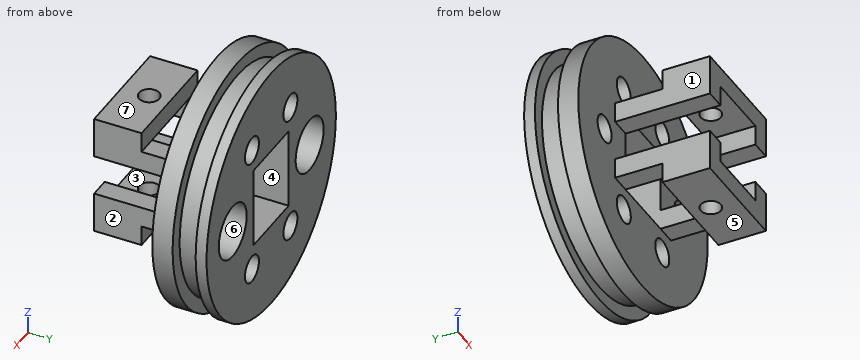
from build123d import *

# Parameters (mm, degrees)
SKETCH_1_R               = 11
EXTRUDE_1_DEPTH          = 9
SKETCH_2_R               = 1
CUT_EXTRUDE_1_DEPTH      = 10
SKETCH_3_R               = 16.549134696
SKETCH_3_R_2             = 9.25
CUT_EXTRUDE_2_DEPTH      = 7
SKETCH_4_W               = 2
SKETCH_4_H               = 1.7
SKETCH_5_W               = 5
SKETCH_5_H               = 6
CUT_EXTRUDE_3_DEPTH      = 7
SKETCH_6_R               = 1.4
CUT_EXTRUDE_4_DEPTH      = 7
PATTERN_CIRCULAR_1_COUNT = 3
PATTERN_CIRCULAR_1_ANGLE = 120
SKETCH_10_R              = 17.755262973
CUT_EXTRUDE_8_DEPTH      = 5
SKETCH_11_R              = 2
CUT_EXTRUDE_9_DEPTH      = 3
SKETCH_12_W              = 1.5
SKETCH_12_H              = 1.5
EXTRUDE_2_DEPTH          = 3.5
SKETCH_14_W              = 1.5
SKETCH_14_H              = 1.5
EXTRUDE_3_DEPTH          = 3.5
SKETCH_13_R              = 0.75
CUT_EXTRUDE_11_DEPTH     = 18.989580318


with BuildPart() as part:
    # 草图1 → 凸台-拉伸1 (new body)
    with BuildSketch(Plane(origin=(0, 0, 0), x_dir=(1, 0, 0), z_dir=(0, 1, 0))):
        with Locations(Location((0, 0, 0), (0, 0, 270))):
            Circle(SKETCH_1_R)
    extrude(amount=EXTRUDE_1_DEPTH)

    # 草图2 → 切除-拉伸1 (cut)
    with BuildSketch(Plane(origin=(0, 9, 0), x_dir=(1, 0, 0), z_dir=(0, 1, 0))):
        with Locations(Location((-5.5, 0, 0), (0, 0, 270))):
            Circle(SKETCH_2_R)
        with Locations(Location((5.5, 0, 0), (0, 0, 270))):
            Circle(SKETCH_2_R)
    cut_extrude_1 = extrude(amount=-CUT_EXTRUDE_1_DEPTH, mode=Mode.SUBTRACT)

    # 草图3 → 切除-拉伸2 (cut)
    with BuildSketch(Plane.XZ):
        Circle(SKETCH_3_R)
        with Locations(Location((0, 0, 0), (0, 0, 270))):
            Circle(SKETCH_3_R_2, mode=Mode.SUBTRACT)
    extrude(amount=-CUT_EXTRUDE_2_DEPTH, mode=Mode.SUBTRACT)

    # 草图4 → 切除-旋转1 (revolve, cut)
    with BuildSketch(Plane.XY, mode=Mode.PRIVATE) as cut_revolve_1_sk:
        with Locations((-9.25, 5.45)):
            Rectangle(SKETCH_4_W, SKETCH_4_H)
        with Locations((-9.25, 2.35)):
            Rectangle(SKETCH_4_W, SKETCH_4_H)
    revolve(cut_revolve_1_sk.sketch.rotate(Axis((0, 0, 0), (0, 1, 0)), 270), axis=Axis((0, 0, 0), (0, 1, 0)), mode=Mode.SUBTRACT)

    # 草图5 → 切除-拉伸3 (cut)
    with BuildSketch(Plane.XZ):
        Rectangle(SKETCH_5_W, SKETCH_5_H)
    extrude(amount=-CUT_EXTRUDE_3_DEPTH, mode=Mode.SUBTRACT)

    # 草图6 → 切除-拉伸4 (cut)
    with BuildSketch(Plane(origin=(0, 9, 0), x_dir=(1, 0, 0), z_dir=(0, 1, 0))):
        with Locations(Location((0, 0, 0), (0, 0, 270))):
            Circle(SKETCH_6_R)
    extrude(amount=-CUT_EXTRUDE_4_DEPTH, mode=Mode.SUBTRACT)

    # 阵列(圆周)1: 切除-拉伸1 ×3 about axis
    pattern_circular_1_axis = Axis((0, 0, 0), (0, -1, 0))
    for i in range(1, PATTERN_CIRCULAR_1_COUNT):
        add(cut_extrude_1.rotate(pattern_circular_1_axis, i * PATTERN_CIRCULAR_1_ANGLE / (PATTERN_CIRCULAR_1_COUNT - 1)), mode=Mode.SUBTRACT)

    # 草图10 → 切除-拉伸8 (cut)
    with BuildSketch(Plane(origin=(0, 9, 0), x_dir=(1, 0, 0), z_dir=(0, 1, 0))):
        Circle(SKETCH_10_R)
    extrude(amount=-CUT_EXTRUDE_8_DEPTH, mode=Mode.SUBTRACT)

    # 草图11 → 切除-拉伸9 (cut)
    with BuildSketch(Plane(origin=(0, 4, 0), x_dir=(1, 0, 0), z_dir=(0, 1, 0))):
        with Locations(Location((-5.5, 0, 0), (0, 0, 270))):
            Circle(SKETCH_11_R)
        with Locations(Location((5.5, 0, 0), (0, 0, 270))):
            Circle(SKETCH_11_R)
    extrude(amount=-CUT_EXTRUDE_9_DEPTH, mode=Mode.SUBTRACT)

    # 草图12 → 凸台-拉伸2 (add)
    with BuildSketch(Plane.XZ):
        with Locations((-3.25, 2.25)):
            Rectangle(SKETCH_12_W, SKETCH_12_H)
        with Locations((3.25, 2.25)):
            Rectangle(SKETCH_12_W, SKETCH_12_H)
        with Locations((3.25, -2.25)):
            Rectangle(SKETCH_12_W, SKETCH_12_H)
        with Locations((-3.25, -2.25)):
            Rectangle(SKETCH_12_W, SKETCH_12_H)
    extrude(amount=EXTRUDE_2_DEPTH)

    # 草图14 → 凸台-拉伸3 (add)
    with BuildSketch(Plane.XZ.offset(3.5)):
        Polygon((-4, 4.5), (-4, 3), (-2.5, 3), (2.5, 3), (2.5, 1.5), (4, 1.5), (4, 4.5), align=None)
        with Locations((-3.25, 2.25)):
            Rectangle(SKETCH_14_W, SKETCH_14_H)
        Polygon((-2.5, -3), (-2.5, -1.5), (-4, -1.5), (-4, -4.5), (4, -4.5), (4, -1.5), (2.5, -1.5), (2.5, -3), align=None)
    extrude(amount=EXTRUDE_3_DEPTH)

    # 草图13 → 切除-拉伸11 (cut, through all)
    with BuildSketch(Plane(origin=(0, 0, 4.5), x_dir=(-1, 0, 0), z_dir=(0, 0, -1))):
        with Locations(Location((0, -5, 0), (0, 0, 180))):
            Circle(SKETCH_13_R)
    extrude(amount=CUT_EXTRUDE_11_DEPTH, mode=Mode.SUBTRACT)


solid = part.part
For this review, take the finished solid that the model builds, in its own axes (mm). Face numbers are marked on the shaded views. A direction names the side the tool comes from. Round coordinates to 2 decimals unless told otherwise and drop trailing zeros. Loops run counter-clockwise (first coordinate to the right, second up) from the corner with the lowest first, then second, coordinate; pieces in that order, holes last. Notation, with made-up numbers: (-10.75, 86.25) - (29.25, 86.25) arc R20 ccw to (29.25, 90.25) - close; hole circle Ø8 at (-8.75, 21.25). An arc over 180 degrees is marked (long way). One line per item, written item: value. Start each with the question number.
Item 1: Take a section at B-B (x = 0). State how many separate pieces and enclosed holes the cut face has, plus the area to 3 significant figures.
Item 2: For L1, parallel to Y at x = 0, z = -3.85; L2, parallel to X at y = 2.8, z = 0; L3, parallel to X at y = -2, z = -2.25, list the stretches that pass through material, from the lowest coordinate up.
Item 3: Take a section at A-A (y = -5). Give the boundary of the cut face in (x, z).
Item 4: The part is to be moulded in two halves that separate along X. For the marked faces 1, 2 and 3, say which applies: +X half, -X half, draft (parallel to the pull), parting line (faces both ways), or undercut.
Item 5: For the marked faces 4, 5, 6 and 7, list the 3-axis set-ups (+Z, -Z, +X, -X, +Y, -Y) from which the entire face can be reached by the end or side of a thin tool; tool diameter is ignored.
Item 6: Take a section at C-C (z = -2.25). Give the boundary of the cut face in (x, y).
Item 7: Clearance check with flat-ended pins moving along their axes: pin 1 Ø0.8 at (x, y) = (3.5, -3) entering from +Z; pin 2 Ø2 at (x, z) = (-5.5, 0.5) entering from +Y; pin 3 Ø3 at (x, y) = (5, -4.5) entering from -Z. State where each tip first meets the part, or that it passes through.
Answer below:
1. separate pieces: 6
1. enclosed holes: 0
1. area: 52.6 mm2
2. L1: y = -7 to -5.75, -4.25 to -3.5, 0 to 4
2. L2: x = -8.25 to -7.5, -3.5 to -2.5, 2.5 to 3.5, 7.5 to 8.25
2. L3: x = -4 to -2.5, 2.5 to 4
3. outline: (-4, -4.5) - (-0.75, -4.5) - (-0.75, -3) - (-2.5, -3) - (-2.5, -1.5) - (-4, -1.5) - close; (-4, 1.5) - (-2.5, 1.5) - (-2.5, 3) - (-0.75, 3) - (-0.75, 4.5) - (-4, 4.5) - close; (0.75, -4.5) - (4, -4.5) - (4, -1.5) - (2.5, -1.5) - (2.5, -3) - (0.75, -3) - close; (0.75, 3) - (2.5, 3) - (2.5, 1.5) - (4, 1.5) - (4, 4.5) - (0.75, 4.5) - close
4. face 1: -X half
4. face 2: +X half
4. face 3: undercut
5. face 4: +Y, -Y
5. face 5: -Z, +X, -X, -Y
5. face 6: +Y
5. face 7: +Z, +X, -X, -Y
6. outline: (-8.97, 0) - (-4, 0) - (-4, -7) - (-2.5, -7) - (-2.5, 4) - (-8.97, 4) - (-8.97, 3.2) - (-7.94, 3.2) - (-7.94, 1.5) - (-8.97, 1.5) - close; (2.5, -7) - (4, -7) - (4, 0) - (8.97, 0) - (8.97, 1.5) - (7.94, 1.5) - (7.94, 3.2) - (8.97, 3.2) - (8.97, 4) - (2.5, 4) - close
7. pin 1: stops at z = 3
7. pin 2: stops at y = 1
7. pin 3: stops at z = -4.5
